Could you check a few things on this drawing? It's one solid part, dimensions in mm from its lowest x, y, z. A direction names the side the tool comes from. Coordinates: 2 decimals unless noted, no trailing zeros. Order: outer loops, then holes, each group sorted by start corner. A loop starts at its lowest first (then second) coordinate and runs counter-clockwise, first axis right, second up. Notation, with made-up numbers: (6, 26.25) -> (10, 26.25) arc R14 ccw to (10, 53.25) -> close; hole circle Ø6 at (13, -39.5). An arc over 180 degrees is marked (long way). Use a Markdown table: item, result. Add a question column.
1. For pin 1 Ø4 at (x, y) = (1, 21) entering from -Z, with a flat end and sliding along its axis, tell me the tip position at first contact or that it passes through.
2. Suppose I cut it at D-D, the plane y = 13.25. List the corners of the cut face in (x, z) for me.
3. Suppose I cut it at A-A, the plane x = 4. List the corners of the cut face in (y, z) for me, then the cut area to 3 significant figures.
4. If I drill on line 1 along Y through (x, z) = (2.25, 5); line 2 along X through (y, z) = (3.5, 5); line 3 along X through (y, z) = (3.75, 0.5), over which ranges is the centre line in solid material (lowest first)? Write a range as from..to.
5. We'd pull the mould along X, two halves only. Please class the marked faces 3, 4 and 5: pulls with the +X half, pulls with the -X half, needs draft (parallel to the pull), parting line crosses it, or undercut.
6. For the marked faces 1 and 2, which set-ups out of +Z, -Z, +X, -X, +Y, -Y let a thin tool reach every point of the face, with its end or its side?
7. Suppose I cut it at B-B, the plane z = 3.5. List the corners of the cut face in (x, y) for me.
8. Suppose I cut it at C-C, the plane y = 4.25. List the corners of the cut face in (x, z) for me, then the cut area to 3 significant figures.
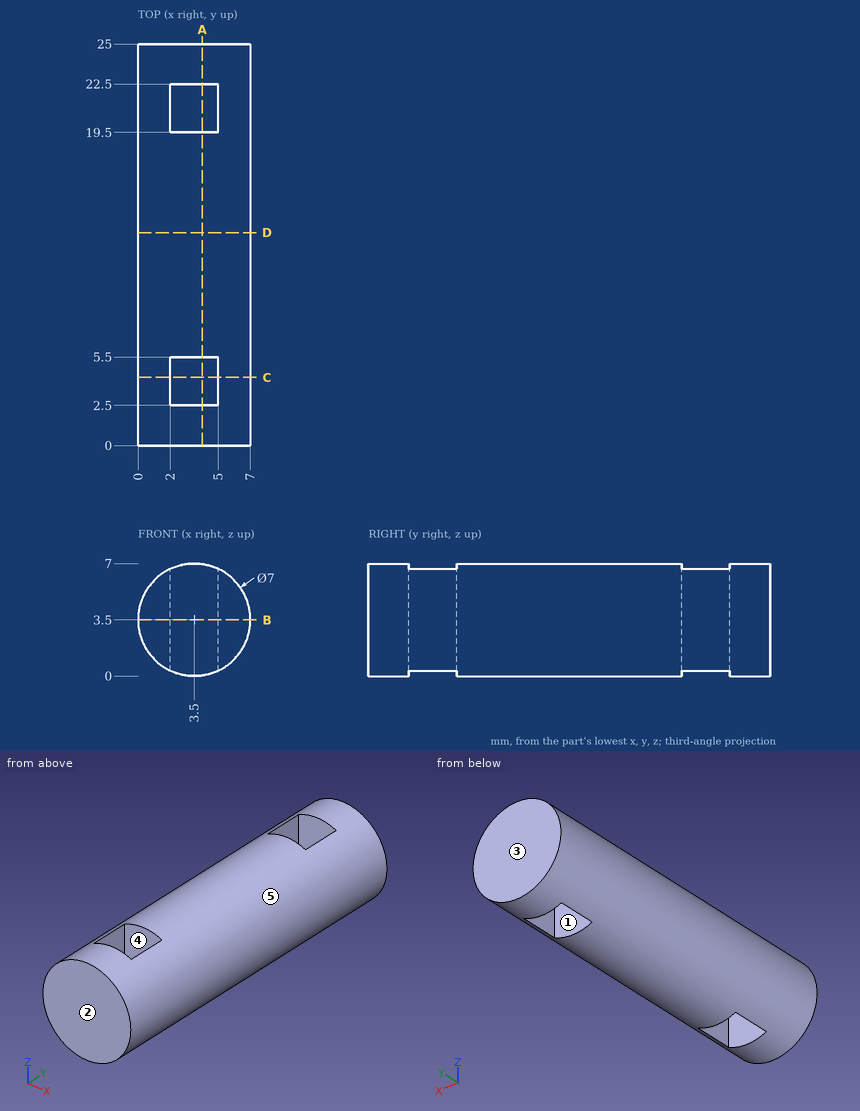
Worked out:
| question | item | result |
|---|---|---|
| 1 | pin 1 | stops at z = 0.2 |
| 2 | outline | circle Ø7 at (3.5, 3.5) |
| 3 | outline | (0, 0.04) -> (2.5, 0.04) -> (2.5, 6.96) -> (0, 6.96) -> close; (5.5, 0.04) -> (19.5, 0.04) -> (19.5, 6.96) -> (5.5, 6.96) -> close; (22.5, 0.04) -> (25, 0.04) -> (25, 6.96) -> (22.5, 6.96) -> close |
| 3 | area | 132 mm² |
| 4 | line 1 | y = 0..2.5, 5.5..19.5, 22.5..25 |
| 4 | line 2 | x = 0.34..2, 5..6.66 |
| 4 | line 3 | x = 1.7..2, 5..5.3 |
| 5 | face 3 | needs draft |
| 5 | face 4 | undercut |
| 5 | face 5 | parting line crosses it |
| 6 | face 1 | +Z, -Z |
| 6 | face 2 | +Z, -Z, +X, -X, -Y |
| 7 | outline | (0, 0) -> (7, 0) -> (7, 25) -> (0, 25) -> close; hole (2, 2.5) -> (5, 2.5) -> (5, 5.5) -> (2, 5.5) -> close; hole (2, 19.5) -> (5, 19.5) -> (5, 22.5) -> (2, 22.5) -> close |
| 8 | outline | (2, 0.34) -> (2, 6.66) arc R3.5 ccw to start; (5, 0.34) arc R3.5 ccw to (5, 6.66) -> close |
| 8 | area | 18.1 mm² |
